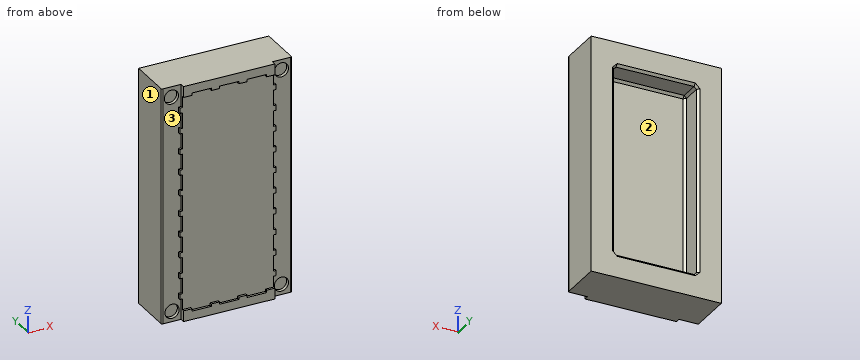
```python
from build123d import *

# Parameters (mm, degrees)
F0_W      = 27.5
F0_H      = 50
F1_DEPTH  = 9.3
F3_DEPTH  = 0.5
F4_R      = 1.5
F5_DEPTH  = 0.75
F6_R      = 0.25
F8_DEPTH  = 0.5
F9_W      = 17.5
F9_H      = 40
F10_DEPTH = 5
F11_SIZE  = 0.5


with BuildPart() as f1:
    # F0 (on Front) → F1 (new body)
    with BuildSketch(Plane.XZ):
        with Locations((13.75, 25)):
            Rectangle(F0_W, F0_H)
    extrude(amount=F1_DEPTH)

    # F2 (on face) → F3 (join)
    with BuildSketch(Plane.XZ.offset(9.3)):
        Polygon((13.75, 50), (4.1195944277, 50), (4.1195944277, 45.3), (3.5795944277, 45.3), (3.5795944277, 44.2), (4.1195944277, 44.2), (4.1195944277, 40.9), (3.5795944277, 40.9), (3.5795944277, 39.8), (4.1195944277, 39.8), (4.1195944277, 36.5), (3.5795944277, 36.5), (3.5795944277, 35.4), (4.1195944277, 35.4), (4.1195944277, 32.1), (3.5795944277, 32.1), (3.5795944277, 31), (4.1195944277, 31), (4.1195944277, 27.7), (3.5795944277, 27.7), (3.5795944277, 26.6), (4.1195944277, 26.6), (4.1195944277, 23.3), (3.5795944277, 23.3), (3.5795944277, 22.2), (4.1195944277, 22.2), (4.1195944277, 18.9), (3.5795944277, 18.9), (3.5795944277, 17.8), (4.1195944277, 17.8), (4.1195944277, 14.5), (3.5795944277, 14.5), (3.5795944277, 13.4), (4.1195944277, 13.4), (4.1195944277, 10.1), (3.5795944277, 10.1), (3.5795944277, 9), (4.1195944277, 9), (4.1195944277, 5.7), (3.5795944277, 5.7), (3.5795944277, 4.6), (4.1195944277, 4.6), (4.1195944277, 0), (13.75, 0), (23.3804055723, 0), (23.3804055723, 4.6), (23.9204055723, 4.6), (23.9204055723, 5.7), (23.3804055723, 5.7), (23.3804055723, 9), (23.9204055723, 9), (23.9204055723, 10.1), (23.3804055723, 10.1), (23.3804055723, 13.4), (23.9204055723, 13.4), (23.9204055723, 14.5), (23.3804055723, 14.5), (23.3804055723, 17.8), (23.9204055723, 17.8), (23.9204055723, 18.9), (23.3804055723, 18.9), (23.3804055723, 22.2), (23.9204055723, 22.2), (23.9204055723, 23.3), (23.3804055723, 23.3), (23.3804055723, 26.6), (23.9204055723, 26.6), (23.9204055723, 27.7), (23.3804055723, 27.7), (23.3804055723, 31), (23.9204055723, 31), (23.9204055723, 32.1), (23.3804055723, 32.1), (23.3804055723, 35.4), (23.9204055723, 35.4), (23.9204055723, 36.5), (23.3804055723, 36.5), (23.3804055723, 39.8), (23.9204055723, 39.8), (23.9204055723, 40.9), (23.3804055723, 40.9), (23.3804055723, 44.2), (23.9204055723, 44.2), (23.9204055723, 45.3), (23.3804055723, 45.3), (23.3804055723, 50), align=None)
    extrude(amount=F3_DEPTH)

    # F4 (on face) → F5 (cut)
    with BuildSketch(Plane.XZ.offset(9.3)):
        with Locations((2.2, 2.2)):
            Circle(F4_R)
        with Locations((25.3, 2.2)):
            Circle(F4_R)
        with Locations((2.0597972139, 47.8)):
            Circle(F4_R)
        with Locations((25.3, 47.8)):
            Circle(F4_R)
    extrude(amount=-F5_DEPTH, mode=Mode.SUBTRACT)

    # F6
    f6_edges = [f1.edges().sort_by_distance(p)[0] for p in [
        (0, -9.3, 25),
        (27.5, -9.3, 25),
    ]]
    fillet(f6_edges, radius=F6_R)

    # F7 (on face) → F8 (join)
    with BuildSketch(Plane.XZ.offset(9.8)):
        Polygon((23.3804055723, 50), (4.1195944277, 50), (4.1195944277, 48.2), (4.1195944277, 47.7), (5.8695944277, 47.7), (5.8695944277, 48.2), (9.9695944277, 48.2), (9.9695944277, 47.7), (11.7195944277, 47.7), (11.7195944277, 48.2), (15.7804055723, 48.2), (15.7804055723, 47.7), (17.5304055723, 47.7), (17.5304055723, 48.2), (21.6304055723, 48.2), (21.6304055723, 47.7), (23.3804055723, 47.7), (23.3804055723, 48.2), align=None)
        Polygon((23.3804055723, 2.3), (21.6304055723, 2.3), (21.6304055723, 1.8), (17.5304055723, 1.8), (17.5304055723, 2.3), (15.7804055723, 2.3), (15.7804055723, 1.8), (11.7195944277, 1.8), (11.7195944277, 2.3), (9.9695944277, 2.3), (9.9695944277, 1.8), (5.8695944277, 1.8), (5.8695944277, 2.3), (4.1195944277, 2.3), (4.1195944277, 1.8), (4.1195944277, 0), (23.3804055723, 0), (23.3804055723, 1.8), align=None)
    extrude(amount=F8_DEPTH)

    # F9 (on face) → F10 (cut)
    with BuildSketch(Plane.XZ):
        with Locations((13.75, 25)):
            Rectangle(F9_W, F9_H)
    extrude(amount=F10_DEPTH, mode=Mode.SUBTRACT)

    # F11
    f11_edges = [f1.edges().sort_by_distance(p)[0] for p in [
        (5, -2.5, 45),
        (13.75, -5, 45),
        (5, -5, 25),
        (22.5, -5, 25),
        (5, -2.5, 5),
        (13.75, -5, 5),
        (22.5, -2.5, 5),
        (13.75, 0, 5),
        (22.5, -2.5, 45),
        (13.75, 0, 45),
        (5, 0, 25),
        (22.5, 0, 25),
    ]]
    chamfer(f11_edges, length=F11_SIZE)


solid = f1.part
```
Verification items for the finished model (mm, model axes). Face numbers are marked on the shaded views. Give positions to 0.01 mm unless a question says otherwise; leave off trailing zeros. Loops run counter-clockwise (first coordinate to the right, second up) from the corner with the lowest first, then second, coordinate; pieces in that order, holes last.
1. Mould release check, pull along X, two halves, no side actions. Record for the marked faces 1, 2 and 3: released by +X, released by -X, zero draft, split by the parting line, or undercut.
2. Go/stop test with a flat-tipped pin: pin 1 Ø5 at (x, z) = (6.5, 39.5) entering from -Y. Record where the tip stops, or that it passes through.
3. Thickness scan on line 1 (Z direction, x = 2.2, y = -8.8); line 2 (Z direction, x = 17, y = -4); line 3 (Y direction, x = 4.25, z = 37.5). Record the ranges inside material, lowest first.
4. Section check C-C, the plane z = 28.5. Enter the section's corners in (x, y), then the cut area to 3 significant figures.
5. Section check D-D, the plane x = 25.3. Enter the section's corners in (y, z).
6. Section check B-B, the plane x = 11.25. Enter the section's corners in (y, z).
7. Section check A-A, the plane y = -2.5. Enter the section's corners in (x, z).
Geometry says:
1. face 1: released by -X
1. face 2: undercut
1. face 3: zero draft
2. pin 1: stops at y = -9.8
3. line 1: z = 0 to 0.7, 3.7 to 46.31, 49.29 to 50
3. line 2: z = 0 to 5, 45 to 50
3. line 3: y = -9.8 to 0
4. outline: (0, -9.05) arc R0.25 ccw to (0.25, -9.3) - (4.12, -9.3) - (4.12, -9.8) - (23.38, -9.8) - (23.38, -9.3) - (27.25, -9.3) arc R0.25 ccw to (27.5, -9.05) - (27.5, 0) - (23, 0) - (22.5, -0.5) - (22.5, -4.5) - (22, -5) - (5.5, -5) - (5, -4.5) - (5, -0.5) - (4.5, 0) - (0, 0) - close
4. area: 178 mm2
5. outline: (-9.3, 0) - (0, 0) - (0, 50) - (-9.3, 50) - (-9.3, 49.3) - (-8.55, 49.3) - (-8.55, 46.3) - (-9.3, 46.3) - (-9.3, 3.7) - (-8.55, 3.7) - (-8.55, 0.7) - (-9.3, 0.7) - close
6. outline: (-10.3, 0) - (0, 0) - (0, 4.5) - (-0.5, 5) - (-4.5, 5) - (-5, 5.5) - (-5, 44.5) - (-4.5, 45) - (-0.5, 45) - (0, 45.5) - (0, 50) - (-10.3, 50) - (-10.3, 47.7) - (-9.8, 47.7) - (-9.8, 2.3) - (-10.3, 2.3) - close
7. outline: (0, 0) - (27.5, 0) - (27.5, 50) - (0, 50) - close; hole (5, 5.5) - (5.5, 5) - (22, 5) - (22.5, 5.5) - (22.5, 44.5) - (22, 45) - (5.5, 45) - (5, 44.5) - close
